Design review of the part shown in the three views and the two pictorial views. Dimensions are in mm from the part's minimum x, y and z. A direction names the side the tool comes from. Round coordinates to 2 decimals unless told otherwise and drop trailing zeros. Write each loop counter-clockwise with the first axis right and the second up, starting at its lowest first coordinate (ties: lowest second). Pieces come first, ordered by that corner, then holes. Notation, with made-up numbers: (-15, 63.25) -> (15, 63.25) arc R18 cw to (15, 89.25) -> close; hole circle Ø10 at (26.5, 19.5). An arc over 180 degrees is marked (long way). One line per question, with ' | ' between items. Start each with the question number.
1) Consider section D-D (z = 3). Give the boundary of the cut face in (x, y) (3 decimals), then the cut area to 3 significant figures.
2) Consider section B-B (z = 26.5). Give the boundary of the cut face in (x, y) (3 decimals).
3) Consider section C-C (y = 4.25). Give the boundary of the cut face in (x, z) (3 decimals).
4) Mouldability with a two-part tool opening along Z and no side actions: class the marked faces 5, 6 and 7 as +Z half, -Z half, draft (parallel to the pull), parting line (faces both ways), or undercut.
5) For probe 1 along Z at (x, y) = (29.5, 2) (3 decimals); probe 2 along X at (y, z) = (1, 24), list the stretches that pass through material, from the lowest coordinate up.
6) Consider section A-A (x = 28.5). Give the boundary of the cut face in (y, z) (3 decimals).
7) Insertion check: pin 1 Ø3 at (x, y) = (4, 3) entering from +Z (3 decimals); pin 2 Ø1.5 at (y, z) = (4.5, 5.5) entering from -X (3 decimals); pin 3 Ø1.9 at (y, z) = (4.5, 27.5) entering from -X. Each pin has a flat end and moves straight along its axis. Give the tip position at first contact, or say it passes through.
8) For the marked faces 1, 2, 3 and 4, list the 3-axis set-ups (+Z, -Z, +X, -X, +Y, -Y) from which the entire face can be reached by the end or side of a thin tool; tool diameter is ignored.
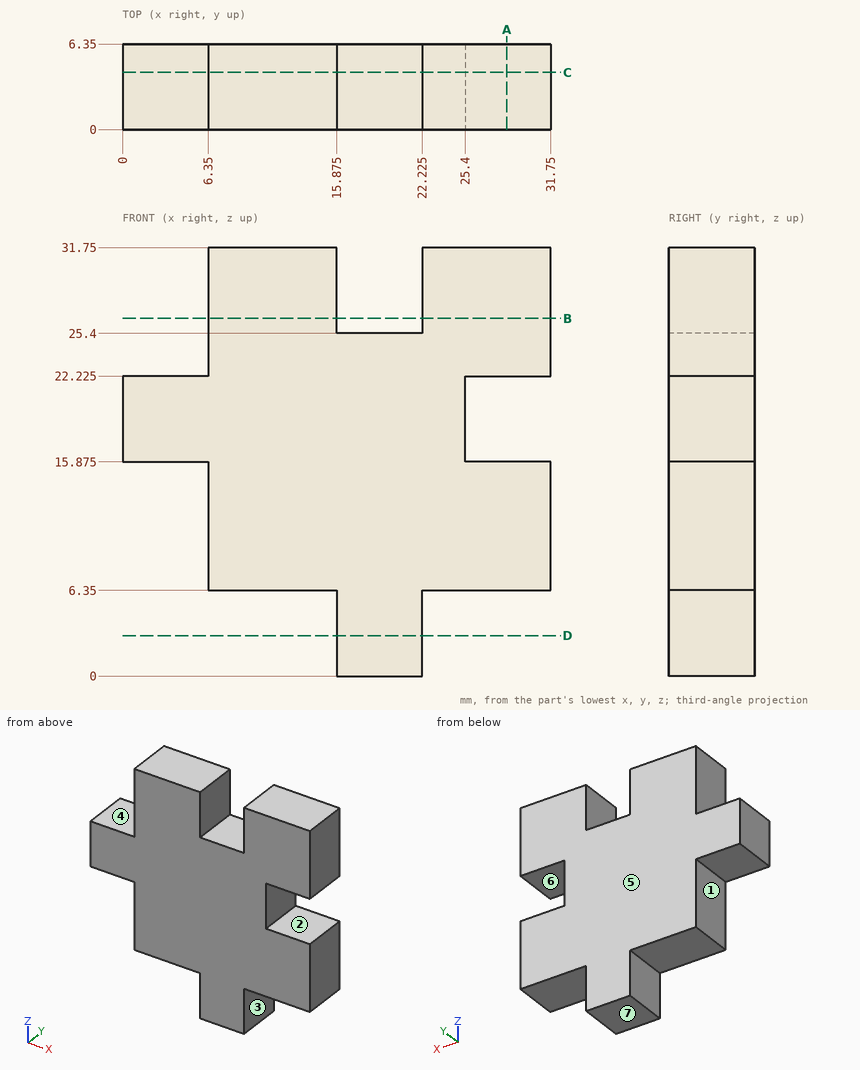
From the geometry:
1) outline: (15.875, 0) -> (22.225, 0) -> (22.225, 6.35) -> (15.875, 6.35) -> close | area: 40.3 mm2
2) outline: (6.35, 0) -> (15.875, 0) -> (15.875, 6.35) -> (6.35, 6.35) -> close; (22.225, 0) -> (31.75, 0) -> (31.75, 6.35) -> (22.225, 6.35) -> close
3) outline: (0, 15.875) -> (6.35, 15.875) -> (6.35, 6.35) -> (15.875, 6.35) -> (15.875, 0) -> (22.225, 0) -> (22.225, 6.35) -> (31.75, 6.35) -> (31.75, 15.875) -> (25.4, 15.875) -> (25.4, 22.225) -> (31.75, 22.225) -> (31.75, 31.75) -> (22.225, 31.75) -> (22.225, 25.4) -> (15.875, 25.4) -> (15.875, 31.75) -> (6.35, 31.75) -> (6.35, 22.225) -> (0, 22.225) -> close
4) face 5: draft | face 6: undercut | face 7: -Z half
5) probe 1: z = 6.35 to 15.875, 22.225 to 31.75 | probe 2: x = 6.35 to 31.75
6) outline: (0, 6.35) -> (6.35, 6.35) -> (6.35, 15.875) -> (0, 15.875) -> close; (0, 22.225) -> (6.35, 22.225) -> (6.35, 31.75) -> (0, 31.75) -> close
7) pin 1: stops at z = 22.225 | pin 2: stops at x = 15.875 | pin 3: stops at x = 6.35
8) face 1: -Z, -X, +Y, -Y | face 2: +X, +Y, -Y | face 3: -Z, +X, +Y, -Y | face 4: +Z, -X, +Y, -Y
